Here's how the part is built. I have some questions about the finished solid (model axes, mm). A direction names the side the tool comes from. Coordinates: 2 decimals unless noted, no trailing zeros. Write each loop counter-clockwise with the first axis right and the second up, starting at its lowest first coordinate (ties: lowest second). Pieces come first, ordered by that corner, then holes. Notation, with made-up numbers: (60.5, 33) -> (79.5, 33) arc R11 ccw to (79.5, 51) -> close; hole circle Ø6 at (55, 47.25). An arc over 180 degrees is marked (long way). Answer in a Markdown table with one row per item. Add a question column.
from build123d import *

# Parameters (mm, degrees)
EXTRUDE_1_DEPTH      = 4
EXTRUDE_2_DEPTH      = 16
SKETCH_3_W           = 170
SKETCH_3_H           = 170
CUT_EXTRUDE_2_DEPTH  = 1
SKETCH_4_W           = 170
SKETCH_4_H           = 170
EXTRUDE_3_DEPTH      = 3
EXTRUDE_4_DEPTH      = 86
SKETCH_7_W           = 10
SKETCH_7_H           = 3
SKETCH_7_W_2         = 3
SKETCH_7_H_2         = 7
SKETCH_7_W_3         = 7
SKETCH_7_H_3         = 10
EXTRUDE_6_DEPTH      = 86
SKETCH_8_R           = 1.5
CUT_EXTRUDE_3_DEPTH  = 86
SKETCH_9_R           = 1.606229087
SKETCH_9_R_2         = 2.055519853
CUT_EXTRUDE_4_DEPTH  = 86
SKETCH_10_W          = 3
SKETCH_10_H          = 3
EXTRUDE_7_DEPTH      = 86
SKETCH_11_R          = 1.5
CUT_EXTRUDE_5_DEPTH  = 86
SKETCH_12_W          = 2
SKETCH_12_H          = 8
EXTRUDE_8_DEPTH      = 86
SKETCH_13_R          = 1.5
CUT_EXTRUDE_6_DEPTH  = 86
SKETCH_14_R          = 3
CUT_EXTRUDE_7_DEPTH  = 2
SKETCH_15_R          = 1.5
CUT_EXTRUDE_8_DEPTH  = 5
SKETCH_16_R          = 3
CUT_EXTRUDE_9_DEPTH  = 2
SKETCH_17_W          = 10
SKETCH_17_H          = 2
SKETCH_17_W_2        = 2
SKETCH_17_H_2        = 10
EXTRUDE_9_DEPTH      = 86
SKETCH_18_R          = 3
CUT_EXTRUDE_10_DEPTH = 2
SKETCH_19_R          = 3
CUT_EXTRUDE_11_DEPTH = 2
SKETCH_22_W          = 20
SKETCH_22_H          = 20
SKETCH_22_R          = 2.6
EXTRUDE_10_DEPTH     = 3


with BuildPart() as part:
    # Sketch 1 → Extrude 1 (new body)
    with BuildSketch(Plane(origin=(0, 0, 0), x_dir=(1, 0, 0), z_dir=(0, 1, 0))):
        Polygon((-80, 62), (-62, 80), (-57, 80), (-57, 85), (57, 85), (57, 80), (62, 80), (80, 62), (80, 57), (85, 57), (85, -57), (80, -57), (80, -62), (62, -80), (57, -80), (57, -85), (-57, -85), (-57, -80), (-62, -80), (-80, -62), (-80, -57), (-85, -57), (-85, 57), (-80, 57), align=None)
    extrude(amount=EXTRUDE_1_DEPTH)

    # Sketch 2 → Extrude 2 (add)
    with BuildSketch(Plane(origin=(0, 4, 0), x_dir=(1, 0, 0), z_dir=(0, 1, 0))):
        Polygon((-57, 85), (57, 85), (57, 80), (62, 80), (80, 62), (80, 57), (85, 57), (85, -57), (80, -57), (80, -62), (62, -80), (57, -80), (57, -85), (-57, -85), (-57, -80), (-62, -80), (-80, -62), (-80, -57), (-85, -57), (-85, 57), (-80, 57), (-80, 62), (-62, 80), (-57, 80), align=None)
        Polygon((-82, 50.757359313), (-50.757359313, 82), (50.757359313, 82), (82, 50.757359313), (82, -50.757359313), (50.757359313, -82), (-50.757359313, -82), (-82, -50.757359313), align=None, mode=Mode.SUBTRACT)
    extrude(amount=EXTRUDE_2_DEPTH)

    # Sketch 3 → Cut-Extrude 2 (cut)
    with BuildSketch(Plane(origin=(0, 0, 0), x_dir=(-1, 0, 0), z_dir=(0, -1, 0))):
        Rectangle(SKETCH_3_W, SKETCH_3_H)
    extrude(amount=-CUT_EXTRUDE_2_DEPTH, mode=Mode.SUBTRACT)

    # Sketch 4 → Extrude 3 (add)
    with BuildSketch(Plane(origin=(0, 20, 0), x_dir=(1, 0, 0), z_dir=(0, 1, 0))):
        Rectangle(SKETCH_4_W, SKETCH_4_H)
        Polygon((82, 50.757359313), (82, -50.757359313), (50.757359313, -82), (-50.757359313, -82), (-82, -50.757359313), (-82, 50.757359313), (-50.757359313, 82), (50.757359313, 82), align=None, mode=Mode.SUBTRACT)
    extrude(amount=EXTRUDE_3_DEPTH)

    # Sketch 5 → Extrude 4 (add)
    with BuildSketch(Plane(origin=(0, 23, 0), x_dir=(1, 0, 0), z_dir=(0, 1, 0))):
        Polygon((85, 85), (-85, 85), (-85, 82), (-82, 82), (-50.757359313, 82), (50.757359313, 82), (85, 82), align=None)
        Polygon((-82, 82), (-85, 82), (-85, -85), (-82, -85), (-82, -50.757359313), (-82, 50.757359313), align=None)
    extrude(amount=EXTRUDE_4_DEPTH)

    # Sketch 7 → Extrude 6 (add)
    with BuildSketch(Plane(origin=(0, 23, 0), x_dir=(1, 0, 0), z_dir=(0, 1, 0))):
        with Locations((-77, -80.5)):
            Rectangle(SKETCH_7_W, SKETCH_7_H)
        with Locations((80.5, -75.5)):
            Rectangle(SKETCH_7_W_2, SKETCH_7_H_2)
        with Locations((80.5, -80.5)):
            Rectangle(SKETCH_7_W_2, SKETCH_7_H)
        with Locations((75.5, -80.5)):
            Rectangle(SKETCH_7_W_3, SKETCH_7_H)
        with Locations((80.5, 77)):
            Rectangle(SKETCH_7_W_2, SKETCH_7_H_3)
    extrude(amount=EXTRUDE_6_DEPTH)

    # Sketch 8 → Cut-Extrude 3 (cut)
    with BuildSketch(Plane.XY.offset(82)):
        with Locations((-77, 86)):
            Circle(SKETCH_8_R)
        with Locations((-77, 46)):
            Circle(SKETCH_8_R)
    extrude(amount=-CUT_EXTRUDE_3_DEPTH, mode=Mode.SUBTRACT)

    # Sketch 9 → Cut-Extrude 4 (cut)
    with BuildSketch(Plane(origin=(82, 0, 0), x_dir=(0, 0, -1), z_dir=(1, 0, 0))):
        with Locations((77, 86)):
            Circle(SKETCH_9_R)
        with Locations((77, 46)):
            Circle(SKETCH_9_R_2)
    extrude(amount=-CUT_EXTRUDE_4_DEPTH, mode=Mode.SUBTRACT)

    # Sketch 10 → Extrude 7 (add)
    with BuildSketch(Plane(origin=(0, 109, 0), x_dir=(1, 0, 0), z_dir=(0, 1, 0))):
        with Locations((80.5, -70.5)):
            Rectangle(SKETCH_10_W, SKETCH_10_H)
        with Locations((70.5, -80.5)):
            Rectangle(SKETCH_10_W, SKETCH_10_H)
    extrude(amount=-EXTRUDE_7_DEPTH)

    # Sketch 11 → Cut-Extrude 5 (cut)
    with BuildSketch(Plane.XY.offset(82)):
        with Locations((74, 86)):
            Circle(SKETCH_11_R)
        with Locations((74, 46)):
            Circle(SKETCH_11_R)
    extrude(amount=-CUT_EXTRUDE_5_DEPTH, mode=Mode.SUBTRACT)

    # Sketch 12 → Extrude 8 (add)
    with BuildSketch(Plane(origin=(0, 109, 0), x_dir=(1, 0, 0), z_dir=(0, 1, 0))):
        with Locations((78, -73)):
            Rectangle(SKETCH_12_W, SKETCH_12_H)
        Polygon((69, -77), (69, -79), (79, -79), (79, -77), (77, -77), align=None)
    extrude(amount=-EXTRUDE_8_DEPTH)

    # Sketch 13 → Cut-Extrude 6 (cut)
    with BuildSketch(Plane.XY.offset(82)):
        with Locations((74, 86)):
            Circle(SKETCH_13_R)
        with Locations((74, 46)):
            Circle(SKETCH_13_R)
    extrude(amount=-CUT_EXTRUDE_6_DEPTH, mode=Mode.SUBTRACT)

    # Sketch 14 → Cut-Extrude 7 (cut)
    with BuildSketch(Plane(origin=(0, 0, 77), x_dir=(-1, 0, 0), z_dir=(0, 0, -1))):
        with Locations((-74, 86)):
            Circle(SKETCH_14_R)
        with Locations((-74, 46)):
            Circle(SKETCH_14_R)
    extrude(amount=-CUT_EXTRUDE_7_DEPTH, mode=Mode.SUBTRACT)

    # Sketch 15 → Cut-Extrude 8 (cut)
    with BuildSketch(Plane(origin=(82, 0, 0), x_dir=(0, 0, -1), z_dir=(1, 0, 0))):
        with Locations((-74, 86)):
            Circle(SKETCH_15_R)
        with Locations((-74, 46)):
            Circle(SKETCH_15_R)
    extrude(amount=-CUT_EXTRUDE_8_DEPTH, mode=Mode.SUBTRACT)

    # Sketch 16 → Cut-Extrude 9 (cut)
    with BuildSketch(Plane.ZY.offset(-77)):
        with Locations((74, 86)):
            Circle(SKETCH_16_R)
        with Locations((74, 46)):
            Circle(SKETCH_16_R)
    extrude(amount=-CUT_EXTRUDE_9_DEPTH, mode=Mode.SUBTRACT)

    # Sketch 17 → Extrude 9 (add)
    with BuildSketch(Plane(origin=(0, 109, 0), x_dir=(1, 0, 0), z_dir=(0, 1, 0))):
        with Locations((-77, -78)):
            Rectangle(SKETCH_17_W, SKETCH_17_H)
        with Locations((78, 77)):
            Rectangle(SKETCH_17_W_2, SKETCH_17_H_2)
    extrude(amount=-EXTRUDE_9_DEPTH)

    # Sketch 18 → Cut-Extrude 10 (cut)
    with BuildSketch(Plane.ZY.offset(-77)):
        with Locations((-77, 86)):
            Circle(SKETCH_18_R)
        with Locations((-77, 46)):
            Circle(SKETCH_18_R)
    extrude(amount=-CUT_EXTRUDE_10_DEPTH, mode=Mode.SUBTRACT)

    # Sketch 19 → Cut-Extrude 11 (cut)
    with BuildSketch(Plane(origin=(0, 0, 77), x_dir=(-1, 0, 0), z_dir=(0, 0, -1))):
        with Locations((77, 86)):
            Circle(SKETCH_19_R)
        with Locations((77, 46)):
            Circle(SKETCH_19_R)
    extrude(amount=-CUT_EXTRUDE_11_DEPTH, mode=Mode.SUBTRACT)

    # Sketch 22 → Extrude 10 (add)
    # profile 1 of 3: a face of its own
    with BuildSketch(Plane(origin=(0, 23, 0), x_dir=(1, 0, 0), z_dir=(0, 1, 0))):
        with Locations((-95, 10)):
            Rectangle(SKETCH_22_W, SKETCH_22_H)
        with Locations(Location((-95, 10, 0), (0, 0, 270))):
            Circle(SKETCH_22_R, mode=Mode.SUBTRACT)
    # profile 2 of 3: a face of its own
    with BuildSketch(Plane(origin=(0, 23, 0), x_dir=(1, 0, 0), z_dir=(0, 1, 0))):
        Polygon((10, -85), (0, -85), (-10, -85), (-10, -105), (0, -105), (10, -105), align=None)
        with Locations(Location((0, -95, 0), (0, 0, 270))):
            Circle(SKETCH_22_R, mode=Mode.SUBTRACT)
    # profile 3 of 3: a face of its own
    with BuildSketch(Plane(origin=(0, 23, 0), x_dir=(1, 0, 0), z_dir=(0, 1, 0))):
        Polygon((85, 10), (85, 0), (85, -10), (105, -10), (105, 0), (105, 10), align=None)
        with Locations(Location((95, 0, 0), (0, 0, 270))):
            Circle(SKETCH_22_R, mode=Mode.SUBTRACT)
    extrude(amount=-EXTRUDE_10_DEPTH)


solid = part.part
Q1. Imagine slicing it at A-A on y = 62. Please give me the cut outline in (x, z), plus the area to 3 significant figures.
Q2. Imagine slicing it at C-C on z = 95. Please give me the cut outline in (x, y).
Q3. If we mould it in two halves opening along Z, with no side actions, what happens to faces 1 (the flat face through (-66.16, 13.37, 66.6)), 2 (the flat face through (-57, 10, -82)), 3 (the flat face through (1, 54, -85))? For each: pulls with the +Z half, pulls with the -Z half, needs draft (parallel to the pull), parting line crosses it, or undercut.
Q4. I need wall thicknesses on line 1 (Y direction, x = 78, z = 74); line 2 (Z direction, x = 81.45, y = 86); line 3 (X direction, y = 22.35, z = 95). Which ranges of each line are inside material? Lowest first, please. Write a range as [from, to].
Q5. I'm going to push flat-ended pins straight in: P1, Ø4, axis at x = -59.5, y = 9.5, coming from the -Z side; P2, Ø5, axis at y = 60.5, z = 65, coming from the -X side; P3, Ø3.5, axis at x = 95.5, y = 22, coming from the -Z side. Where does each tip first touch, or does it pass through?
Q6. Imagine slicing it at B-B on x = 0. Please give me the cut outline in (y, z).
Q7. Imagine slicing it at D-D on x = 95. Please give me the cut outline in (y, z).
Q8. For faces 4 (the flat face through (-66.6, 13.37, -66.16)), 5 (the flat face through (82, 67, 76)), 6 (the flat face through (-71, 10, 71)), 7 (the cylindrical face through (77.99, 48.03, -79.21)), 8 (the flat face through (74, 20, 74)), which set-ups out of +Z, -Z, +X, -X, +Y, -Y let a thin tool reach every point of the face, with its end or its side?
Result sheet:
| question | item | result |
|---|---|---|
| 1 | outline | (-85, -85) -> (85, -85) -> (85, -82) -> (82, -82) -> (82, -72) -> (77, -72) -> (77, -82) -> (-82, -82) -> (-82, 77) -> (-72, 77) -> (-72, 82) -> (-82, 82) -> (-82, 85) -> (-85, 85) -> close; (69, 77) -> (77, 77) -> (77, 69) -> (82, 69) -> (82, 82) -> (69, 82) -> close |
| 1 | area | 1,220 mm^2 |
| 2 | outline | (-10, 20) -> (-2.6, 20) -> (-2.6, 23) -> (-10, 23) -> close; (2.6, 20) -> (10, 20) -> (10, 23) -> (2.6, 23) -> close |
| 3 | face 1 | undercut |
| 3 | face 2 | needs draft |
| 3 | face 3 | pulls with the -Z half |
| 4 | line 1 | y = [20, 43], [49, 83], [89, 109] |
| 4 | line 2 | z = [-85, -78.61], [-75.39, -72], [69, 72.5], [75.5, 82] |
| 4 | line 3 | x = [-10, -2.6], [2.6, 10] |
| 5 | P1 | stops at z = -80 |
| 5 | P2 | stops at x = -85 |
| 5 | P3 | stops at z = -10 |
| 6 | outline | (1, -85) -> (109, -85) -> (109, -82) -> (4, -82) -> (4, 82) -> (23, 82) -> (23, 92.4) -> (20, 92.4) -> (20, 85) -> (1, 85) -> close; (20, 97.6) -> (23, 97.6) -> (23, 105) -> (20, 105) -> close |
| 7 | outline | (20, -10) -> (23, -10) -> (23, -2.6) -> (20, -2.6) -> close; (20, 2.6) -> (23, 2.6) -> (23, 10) -> (20, 10) -> close |
| 8 | face 4 | +Y |
| 8 | face 5 | +Z, +X, +Y |
| 8 | face 6 | +Z, -X, -Y |
| 8 | face 7 | none |
| 8 | face 8 | +Z, +X, -Y |
